Could you check a few things on this drawing? It's one solid part, dimensions in mm from its lowest x, y, z. Round coordinates to 2 decimals unless told otherwise and drop trailing zeros. Loops run counter-clockwise (first coordinate to the right, second up) from the corner with the lowest first, then second, coordinate; pieces in that order, holes last. Notation, with made-up numbers: (85, -5.5) -> (144, -5.5) arc R25 cw to (144, 18.5) -> close; hole circle Ø10 at (-10, -9). An arc over 180 degrees is marked (long way). Write each question's results on one line, items separated by ' | '.
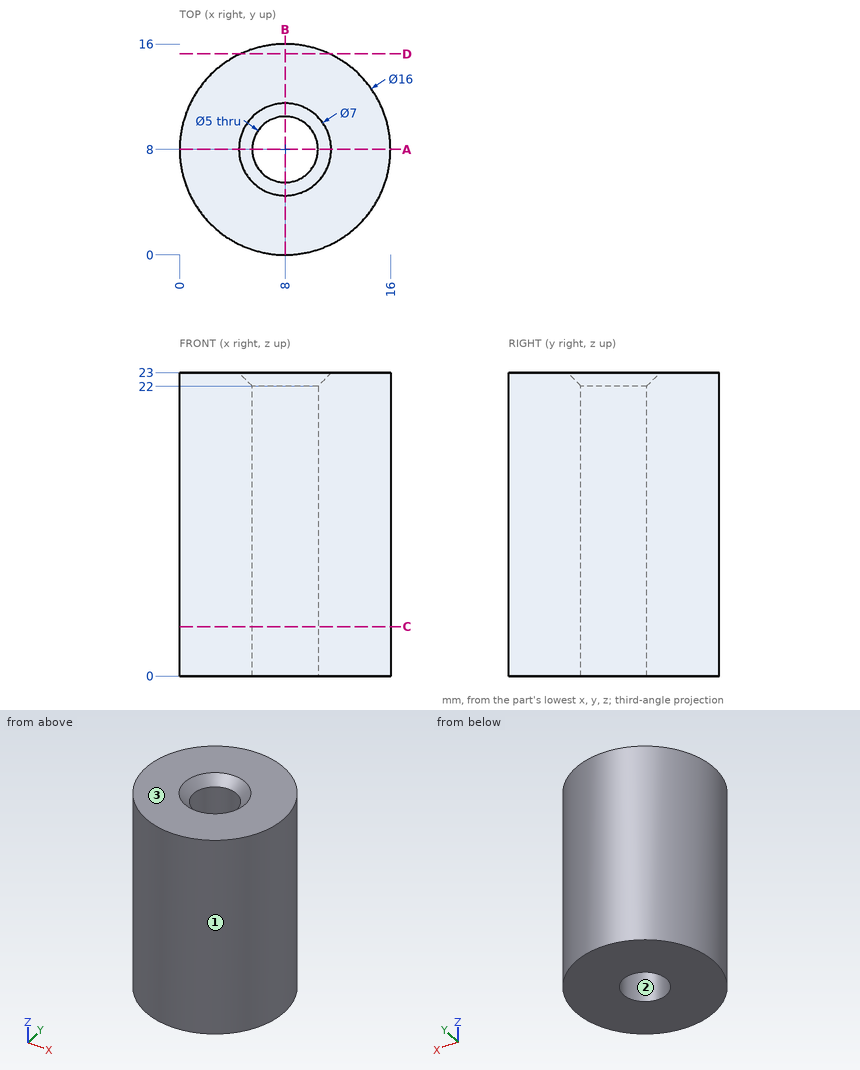
1) I need wall thicknesses on line 1 (Y direction, x = 8, z = 14.5); line 2 (X direction, y = 8.5, z = 4); line 3 (X direction, y = 10, z = 15.5). Which ranges of each line are inside material? Lowest first, please.
Model answer:
line 1: y = 0 to 5.5, 10.5 to 16 | line 2: x = 0.02 to 5.55, 10.45 to 15.98 | line 3: x = 0.25 to 6.5, 9.5 to 15.75
2) I want a section at A-A, the plane y = 8. Write out the boundary of the cut face in (x, z), plus the area to 3 significant figures.
Model answer:
outline: (0, 0) -> (5.5, 0) -> (5.5, 22) -> (4.5, 23) -> (0, 23) -> close; (10.5, 0) -> (16, 0) -> (16, 23) -> (11.5, 23) -> (10.5, 22) -> close | area: 252 mm2
3) I want a section at C-C, the plane z = 3.75. Write out the boundary of the cut face in (x, y).
Model answer:
outline: circle Ø16 at (8, 8); hole circle Ø5 at (8, 8)
4) I want a section at D-D, the plane y = 15.25. Write out the boundary of the cut face in (x, z).
Model answer:
outline: (4.62, 0) -> (11.38, 0) -> (11.38, 23) -> (4.62, 23) -> close
5) I'm going to push flat-ended pins straight in: pin 1 (6 mm diameter, centred on x = 13, z = 16, fed in from -Y); pin 2 (6 mm diameter, centred on x = 4.5, z = 17.5, fed in from -Y); pin 3 (4 mm diameter, centred on x = 8, y = 8, fed in from -Z); pin 4 (8 mm diameter, centred on x = 13, z = 17.5, fed in from +Y). Where does each tip first touch, or does it pass through?
Model answer:
pin 1: stops at y = 0.25 | pin 2: stops at y = 0.02 | pin 3: passes through | pin 4: stops at y = 15.94
6) If we mould it in two halves opening along Y, with no side actions, what happens to the marked faces 1, 2 and 3? For each: released by +Y, released by -Y, zero draft, split by the parting line, or undercut.
Model answer:
face 1: split by the parting line | face 2: undercut | face 3: zero draft
